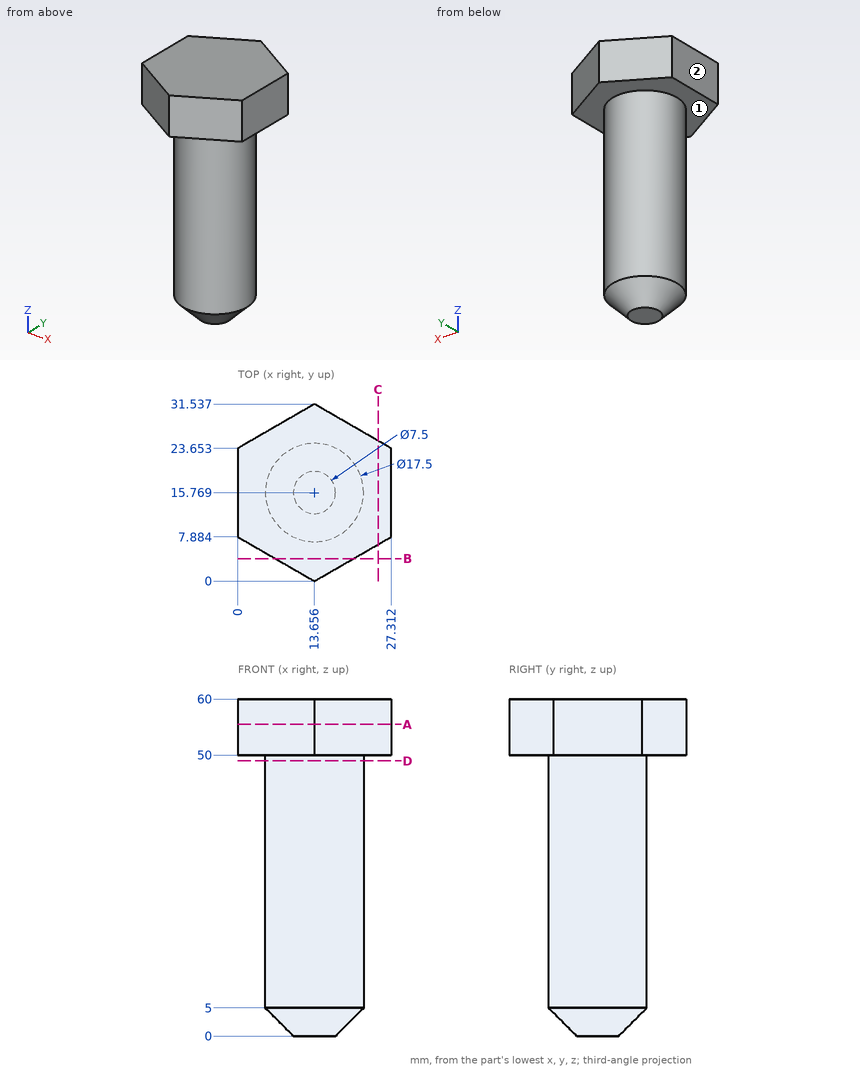
Drawing for the job (mm, zero at the part's lowest x, y, z). A direction names the side the tool comes from. Round coordinates to 2 decimals unless told otherwise and drop trailing zeros. Loops run counter-clockwise (first coordinate to the right, second up) from the corner with the lowest first, then second, coordinate; pieces in that order, holes last. Notation, with made-up numbers: (43.25, 6) -> (65.25, 6) arc R26 cw to (65.25, 44) -> close; hole circle Ø11 at (60, -3.75). An arc over 180 degrees is marked (long way). Use one line per item in the form item = value. Start each with the question number.
Item 1: Band-saw the part on D-D (z = 49). List the corners of the cut face in (x, y).
Item 2: Band-saw the part on B-B (y = 4). List the corners of the cut face in (x, z), plus the area to 3 significant figures.
Item 3: Drill centre lines: line 1 along Z through (x, y) = (17, 27.5); line 2 along Y through (x, z) = (13.75, 25); line 3 along X through (y, z) = (13.5, 21.5) (1 decimal). Where is each one in solid material? Low to high.
Item 4: Band-saw the part on C-C (x = 25). List the corners of the cut face in (y, z), plus the area to 3 significant figures.
Item 5: Tool access for the marked faces 1 and 2: list every direction of +Z, -Z, +X, -X, +Y, -Y with a clear straight run to the whole face (end or side of a thin tool).
Item 6: Band-saw the part on A-A (z = 55.5). List the corners of the cut face in (x, y) (1 decimal), plus the area to 3 significant figures.
Item 7: Drop flat-ended pins along their axis: pin 1 Ø2 at (y, z) = (19.5, 11) entering from +X; pin 2 Ø2 at (x, z) = (18.5, 14) entering from +Y; pin 3 Ø3 at (x, y) = (22, 26) entering from -Z. Give the stop position or say it passes through.
Data:
q1.outline = circle Ø17.5 at (13.66, 15.77)
q2.outline = (6.73, 50) -> (20.58, 50) -> (20.58, 60) -> (6.73, 60) -> close
q2.area = 139 mm^2
q3.line_1 = 50 to 60
q3.line_2 = 7.02 to 24.52
q3.line_3 = 5.2 to 22.1
q4.outline = (6.55, 50) -> (24.99, 50) -> (24.99, 60) -> (6.55, 60) -> close
q4.area = 184 mm^2
q5.face_1 = -Z
q5.face_2 = +Z, -Z, -X, +Y, -Y
q6.outline = (0, 7.9) -> (13.7, 0) -> (27.3, 7.9) -> (27.3, 23.7) -> (13.7, 31.5) -> (0, 23.7) -> close
q6.area = 646 mm^2
q7.pin_1 = 21.97
q7.pin_2 = 23.63
q7.pin_3 = 50
